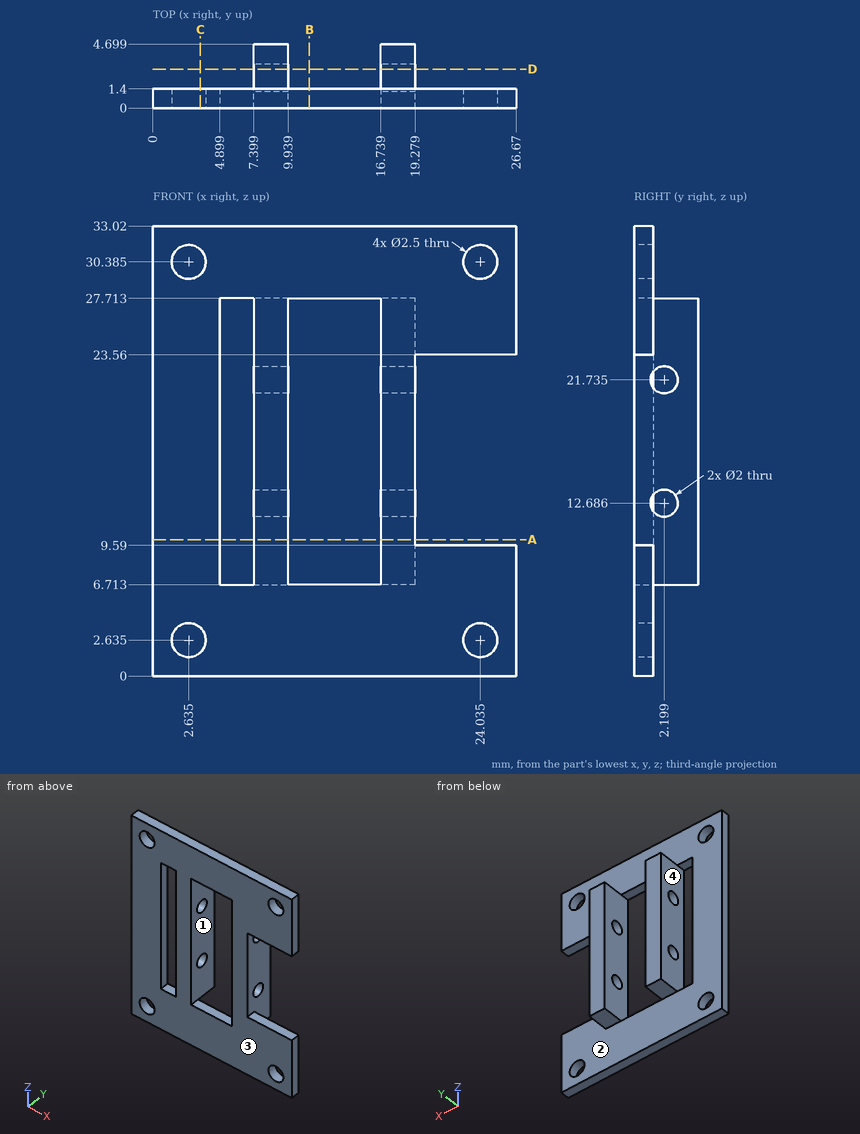
Part print with two shaded views. Sizes in mm from the minimum x, y, z corner. A direction names the side the tool comes from. Coordinates: 2 decimals unless noted, no trailing zeros. Order: outer loops, then holes, each group sorted by start corner. A loop starts at its lowest first (then second) coordinate and runs counter-clockwise, first axis right, second up. Notation, with made-up numbers: (14, 88.25) - (29, 88.25) arc R21 cw to (29, 114.25) - close; hole circle Ø1 at (-23.75, 13). An arc over 180 degrees is marked (long way). Answer in a Markdown table with one row per item.
1. Slice it at A-A, the plane z = 10. List the corners of the cut face in (x, y).
Answer:
| item | result |
|---|---|
| outline | (0, 0) - (4.9, 0) - (4.9, 1.4) - (0, 1.4) - close; (7.4, 0) - (9.94, 0) - (9.94, 4.7) - (7.4, 4.7) - close; (16.74, 0) - (19.28, 0) - (19.28, 4.7) - (16.74, 4.7) - close |
2. Slice it at C-C, the plane x = 3.5. List the corners of the cut face in (y, z).
Answer:
| item | result |
|---|---|
| outline | (0, 0) - (1.4, 0) - (1.4, 1.73) - (0, 1.73) - close; (0, 3.54) - (1.4, 3.54) - (1.4, 29.48) - (0, 29.48) - close; (0, 31.29) - (1.4, 31.29) - (1.4, 33.02) - (0, 33.02) - close |
3. 3-axis set-ups, long thin cutter, end or side, ignore diameter. For the marked faces 3 and 4: which of +Z, -Z, +X, -X, +Y, -Y reach the whole face in a straight line?
Answer:
| item | result |
|---|---|
| face 3 | +Z, -Z, +X, -X, -Y |
| face 4 | +Y, -Y |
4. Flat gauge pins, fed straight in: P1, Ø2.5, axis at y = 2.2, z = 12.69, coming from the +X side; P2, Ø0.8, axis at x = 8, y = 2.5, coming from the -Z side; P3, Ø2.5, axis at y = 3, z = 21.5, coming from the -X side. Where does each tip first touch, or does it go through?
Answer:
| item | result |
|---|---|
| P1 | x = 19.28 |
| P2 | z = 6.71 |
| P3 | x = 7.4 |
5. Pull direction X, two halves, no side cores. Call the marked faces 1 and 2: +X half, -X half, draft (parallel to the pull), parting line (faces both ways), or undercut.
Answer:
| item | result |
|---|---|
| face 1 | undercut |
| face 2 | draft |
6. Slice it at D-D, the plane y = 2.85. List the corners of the cut face in (x, z) (1 decimal).
Answer:
| item | result |
|---|---|
| outline | (7.4, 6.7) - (9.9, 6.7) - (9.9, 11.9) - (7.4, 11.9) - close; (7.4, 13.4) - (9.9, 13.4) - (9.9, 21) - (7.4, 21) - close; (7.4, 22.5) - (9.9, 22.5) - (9.9, 27.7) - (7.4, 27.7) - close; (16.7, 6.7) - (19.3, 6.7) - (19.3, 11.9) - (16.7, 11.9) - close; (16.7, 13.4) - (19.3, 13.4) - (19.3, 21) - (16.7, 21) - close; (16.7, 22.5) - (19.3, 22.5) - (19.3, 27.7) - (16.7, 27.7) - close |
7. Slice it at B-B, the plane x = 11.5. List the corners of the cut face in (y, z).
Answer:
| item | result |
|---|---|
| outline | (0, 0) - (1.4, 0) - (1.4, 6.71) - (0, 6.71) - close; (0, 27.71) - (1.4, 27.71) - (1.4, 33.02) - (0, 33.02) - close |
8. Drill centre lines: L1, parallel to X at y = 0.4, z = 20; L2, parallel to X at y = 0.65, z = 26.5; L3, parallel to X at y = 2.25, z = 24. Where is each one in solid material? Low to high. Write a range as from..to.
Answer:
| item | result |
|---|---|
| L1 | 0..4.9, 7.4..9.94, 16.74..19.28 |
| L2 | 0..4.9, 7.4..9.94, 16.74..26.67 |
| L3 | 7.4..9.94, 16.74..19.28 |
